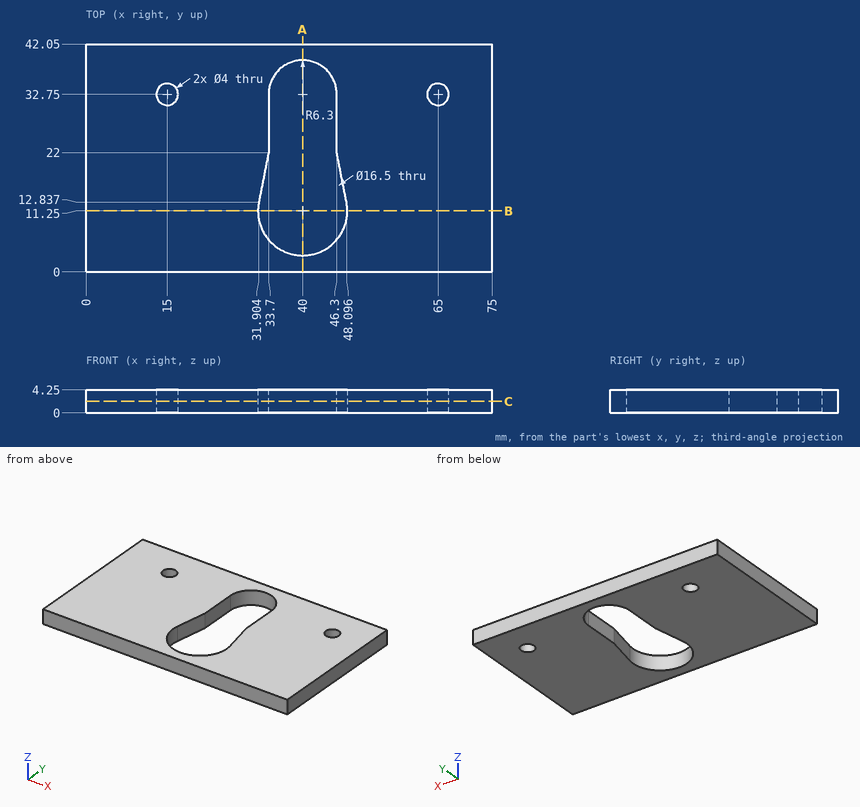
For this review, use the dimensioned drawing (mm, ordinates from the lowest corner) and the shaded views. Give positions to 0.01 mm unless a question says otherwise; leave off trailing zeros. Write each loop counter-clockwise with the first axis right and the second up, starting at its lowest first coordinate (ties: lowest second). Pieces come first, ordered by that corner, then holes. Notation, with made-up numbers: M -30.75,35.25 L 19.25,35.25 A20 ccw 19.25,61.25 Z; hole C 57,7 d8. An arc over 180 degrees is marked long. Answer as a JSON object with one key per item and string values. Group by question number.
1) We need section B-B (y = 11.25). Give the boundary of the cut face in (x, z), and give its area (3 significant figures).
2) We need section C-C (z = 2.1). Give the boundary of the cut face in (x, y), and give its area (3 significant figures).
3) We need section A-A (x = 40). Give the boundary of the cut face in (y, z).
4) For line 1 along Y through (x, z) = (65, 2.2); line 2 along X through (y, z) = (26, 2.9); line 3 along X through (y, z) = (11.5, 3.35), list the stretches that pass through material, from the lowest coordinate up.
Answer key:
{
 "1": {"outline": "M 0,0 L 31.75,0 L 31.75,4.25 L 0,4.25 Z; M 48.25,0 L 75,0 L 75,4.25 L 48.25,4.25 Z", "area": "249 mm²"},
 "2": {"outline": "M 0,0 L 75,0 L 75,42.05 L 0,42.05 Z; hole C 15,32.75 d4; hole M 31.9,12.84 A8.25 ccw long 48.1,12.84 L 46.3,22 L 46.3,32.75 A6.3 ccw 33.7,32.75 L 33.7,22 Z; hole C 65,32.75 d4", "area": "2,670 mm²"},
 "3": {"outline": "M 0,0 L 3,0 L 3,4.25 L 0,4.25 Z; M 39.05,0 L 42.05,0 L 42.05,4.25 L 39.05,4.25 Z"},
 "4": {"line 1": "y = 0 to 30.75, 34.75 to 42.05", "line 2": "x = 0 to 33.7, 46.3 to 75", "line 3": "x = 0 to 31.75, 48.25 to 75"}
}
